Geometry: final body of the model. Coordinates: model frame, mm. A direction names the side the tool comes from. Round coordinates to 2 decimals unless told otherwise and drop trailing zeros. Write each loop counter-clockwise with the first axis right and the second up, starting at its lowest first coordinate (ties: lowest second). Pieces come first, ordered by that corner, then holes. Notation, with made-up numbers: M 58,33.25 L 89,33.25 A36 ccw 89,67.25 Z; hole C 63.25,27 d1. An arc over 180 degrees is marked long. Use one line per item in the form item = value. Start each with the question number.
from build123d import *

# Parameters (mm, degrees)
SKETCH1_W            = 15
SKETCH1_H            = 40
BOSS_EXTRUDE1_DEPTH  = 6
BOSS_EXTRUDE3_DEPTH  = 15
BOSS_EXTRUDE7_DEPTH  = 15
BOSS_EXTRUDE9_DEPTH  = 15
BOSS_EXTRUDE10_DEPTH = 15
BOSS_EXTRUDE11_DEPTH = 15
CUT_EXTRUDE2_REACH   = 87
SKETCH11_R           = 2


with BuildPart() as part:
    # Sketch1 → Boss-Extrude1 (new body)
    with BuildSketch(Plane(origin=(0, 0, 0), x_dir=(1, 0, 0), z_dir=(0, 1, 0))):
        with Locations((7.5, 20)):
            Rectangle(SKETCH1_W, SKETCH1_H)
    extrude(amount=BOSS_EXTRUDE1_DEPTH)

    # Sketch2 → Boss-Extrude3 (add)
    with BuildSketch(Plane.ZY):
        with BuildLine():
            Line((0, 0), (0, 6))
            ThreePointArc((0, 6), (23.660865618, -36.5), (0, -79))
            ThreePointArc((0, -79), (14.836408469, -39.5), (0, 0))
        make_face()
    extrude(amount=-BOSS_EXTRUDE3_DEPTH)

    # Sketch4 → Boss-Extrude7 (add)
    with BuildSketch(Plane.ZY):
        with BuildLine():
            ThreePointArc((2.687694394, -75.697436861), (-4.903747344, -32.637432794), (-34, 0))
            Line((-34, 0), (-40, 0))
            ThreePointArc((-40, 0), (-9.691402152, -34.280456786), (0, -79))
            ThreePointArc((0, -79), (1.37315296, -77.372568069), (2.687694394, -75.697436861))
        make_face()
    extrude(amount=-BOSS_EXTRUDE7_DEPTH)

    # Sketch6 → Boss-Extrude9 (add)
    with BuildSketch(Plane(origin=(15, 0, 0), x_dir=(0, 0, -1), z_dir=(1, 0, 0))):
        with BuildLine():
            Line((-23.598326506, -39), (6.336124845, -29.82478781))
            ThreePointArc((6.336124845, -29.82478781), (7.039786657, -35.139310612), (2.528857435, -38.036000122))
            Line((2.528857435, -38.036000122), (-23.598326506, -39))
        make_face()
    extrude(amount=-BOSS_EXTRUDE9_DEPTH)

    # Sketch7 → Boss-Extrude10 (add)
    with BuildSketch(Plane(origin=(15, 0, 0), x_dir=(0, 0, -1), z_dir=(1, 0, 0))):
        Polygon((-12.974883891, -54.329621557), (5.491788936, -43.926999792), (-14.212166694, -65.750503945), align=None)
    extrude(amount=-BOSS_EXTRUDE10_DEPTH)

    # Sketch8 → Boss-Extrude11 (add)
    with BuildSketch(Plane(origin=(15, 0, 0), x_dir=(0, 0, -1), z_dir=(1, 0, 0))):
        Polygon((-15.593532308, -9.266721382), (6.336124845, -29.82478781), (2.528857435, -38.036000122), align=None)
    extrude(amount=-BOSS_EXTRUDE11_DEPTH)

    # Sketch11 → Cut-Extrude2 (cut, up to next)
    with BuildSketch(Plane(origin=(0, 6, 0), x_dir=(1, 0, 0), z_dir=(0, 1, 0)), mode=Mode.PRIVATE) as cut_extrude2_sk1:
        with Locations((7.5, 26)):
            Circle(SKETCH11_R)
    cut_extrude2_tool1 = extrude(cut_extrude2_sk1.sketch, amount=-CUT_EXTRUDE2_REACH, mode=Mode.PRIVATE) & part.part
    add(cut_extrude2_tool1.solids().sort_by_distance((7.5, 6, -26))[0], mode=Mode.SUBTRACT)
    # Sketch11 → Cut-Extrude2 (cut, up to next)
    with BuildSketch(Plane(origin=(0, 6, 0), x_dir=(1, 0, 0), z_dir=(0, 1, 0)), mode=Mode.PRIVATE) as cut_extrude2_sk2:
        with Locations((7.5, 14)):
            Circle(SKETCH11_R)
    cut_extrude2_tool2 = extrude(cut_extrude2_sk2.sketch, amount=-CUT_EXTRUDE2_REACH, mode=Mode.PRIVATE) & part.part
    add(cut_extrude2_tool2.solids().sort_by_distance((7.5, 6, -14))[0], mode=Mode.SUBTRACT)


solid = part.part
1. Section query A-A (x = 7.5). Return loops of the section in (y, z), then the cut area to 3 significant figures.
2. Section query C-C (z = -14). Return loops of the section in (x, y).
3. Set-up query: faces 1 (the face through (0, -24, 1)), 2 (the face through (6.026, 3.042, -15.352)), 3 (the face through (7.6, -50.87, 6.83)). Return all of +Z, -Z, +X, -X, +Y, -Y with unobstructed straight access to the full face (end or side cutting, diameter ignored); none if empty.
4. Contact query for flat-ended pins moving along their axis: pin 1 (5 mm diameter, centred on x = 11.5, y = -57, fed in from -Z); pin 2 (1.5 mm diameter, centred on x = 11, z = 10.5, fed in from +Y); pin 3 (2 mm diameter, centred on x = 12, z = 2, fed in from -Y). Output: stop coordinate, or through.
5. Ray query, probe 1 along X at (y, z) = (4.75, -26); probe 2 along Z at (x, y) = (7.5, 3.65); probe 3 along Y at (x, z) = (12, 8). Return the intervals inside material, ascending.
6. Section query B-B (z = -30). Return loops of the section in (x, y).
7. Section query D-D (y = -56). Return loops of the section in (x, z).
8. Pull-direction query (Z, two-part tool) for faces 4 (the face through (7.066, 3.042, -24.048)), 5 (the face through (7.395, -35.789, 23.656)), 6 (the face through (7.4, -33.7, -9.99)); classes: released by +Z, released by -Z, zero draft, split by the parting line, or undercut.
Checks:
q1.outline = M -79,0 A90.6 cw 0,-40 L 6,-40 L 6,-28 L 0,-28 L 0,-34 A80 ccw -29.82,-6.34 L -14.92,9.57 A60 cw 0,0 L 0,-12 L 6,-12 L 6,0 A50 ccw Z; M 0,-24 L 6,-24 L 6,-16 L 0,-16 Z; hole M -75.7,2.69 A80 cw -51.7,1.52 L -61.72,10.57 A60 ccw Z; hole M -54.33,12.97 L -47.31,0.51 A80 cw -38.04,-2.53 L -38.68,14.83 A60 ccw Z; hole M -36.29,14.75 L -32.13,1.19 L -17.26,10.56 A60 ccw Z
q1.area = 1,460 mm^2
q2.outline = M 0,-26.7 L 15,-26.7 L 15,-18.09 L 0,-18.09 Z; M 0,0 L 5.5,0 L 5.5,6 L 0,6 Z; M 9.5,0 L 15,0 L 15,6 L 9.5,6 Z
q3.face_1 = +Z, -Z, -X, +Y, -Y
q3.face_2 = +Y
q3.face_3 = +X, -X
q4.pin_1 = -2.32
q4.pin_2 = -1.89
q4.pin_3 = -78.36
q5.probe_1 = 0 to 5.5, 9.5 to 15
q5.probe_2 = -40 to -28, -24 to -16, -12 to 3.46
q5.probe_3 = -72.84 to -67.31, -58.87 to -51.53, -38.42 to -34.22, -21.32 to -16.39, -11.69 to -0.16
q6.outline = M 0,-7.79 L 15,-7.79 L 15,-2.71 L 0,-2.71 Z; M 0,0 L 15,0 L 15,6 L 0,6 Z
q7.outline = M 0,-1.98 L 15,-1.98 L 15,2.27 L 0,2.27 Z; M 0,5.41 L 15,5.41 L 15,19.7 L 0,19.7 Z
q8.face_4 = undercut
q8.face_5 = released by +Z
q8.face_6 = released by -Z
